```python
from build123d import *

# Parameters (mm, degrees)
F0_R     = 74.736194
F1_DEPTH = 25.4
F2_SIZE  = 5.08


with BuildPart() as f1:
    # F0 (on Top) → F1 (new body)
    with BuildSketch(Plane.XY):
        with Locations((-20.023532, 0)):
            Circle(F0_R)
        Polygon((-49.93894, 17.944667), (-38.893249, 41.878957), (14.034008, 41.878957), (0, 12.881645), (13.113534, 12.881645), (-11.739265, -19.337591), (7.130454, -19.337591), (-38.893249, -57.080124), (-29.228272, -17.496489), (-49.93894, -17.496489), (-31.529456, 17.944667), align=None, mode=Mode.SUBTRACT)
    extrude(amount=F1_DEPTH)

    # F2
    f2_edges = [f1.edges().sort_by_distance(p)[0] for p in [
        (-94.759726, 0, 25.4),
    ]]
    chamfer(f2_edges, length=F2_SIZE)


solid = f1.part
```
Design review of the part built by this model. Coordinates are the model's own, in mm. A direction names the side the tool comes from. Coordinates: 2 decimals unless noted, no trailing zeros. Order: outer loops, then holes, each group sorted by start corner. A loop starts at its lowest first (then second) coordinate and runs counter-clockwise, first axis right, second up. Notation, with made-up numbers: (24.25, 70) - (53.25, 70) arc R18 cw to (53.25, 104) - close; hole circle Ø7 at (16, 0.25). An arc over 180 degrees is marked (long way). Answer in a Markdown table with one row per item.
(1) Consider section A-A on z = 13.75. State the section outline as (x, y) points.
Checked values:
| item | result |
|---|---|
| outline | circle Ø149.47 at (-20.02, 0); hole (-49.94, -17.5) - (-29.23, -17.5) - (-38.89, -57.08) - (7.13, -19.34) - (-11.74, -19.34) - (13.11, 12.88) - (0, 12.88) - (14.03, 41.88) - (-38.89, 41.88) - (-49.94, 17.94) - (-31.53, 17.94) - close |
(2) Wall thickness on line 1 along Y through (x, z) = (-10, 8.25); line 2 along Y through (x, z) = (9, 11.75); line 3 along X through (y, z) = (21, 20.25): over which ranges is each line inside the solid? List them lowest first. Write a range as from..to.
Checked values:
| item | result |
|---|---|
| line 1 | -74.06..-33.39, -19.34..-17.08, 41.88..74.06 |
| line 2 | -68.87..7.55, 12.88..31.48, 41.88..68.87 |
| line 3 | -91.75..-48.53, 3.93..51.7 |
(3) Clearance check with flat-ended pins moving along their axes: pin 1 (1 mm diameter, centred on y = -14.5, z = 14.5, fed in from -X); pin 2 (14.5 mm diameter, centred on x = -43.5, z = 11, fed in from +Y); pin 3 (1 mm diameter, centred on y = 24, z = 9, fed in from -X). State where each tip first meets the part, or that it passes through.
Checked values:
| item | result |
|---|---|
| pin 1 | x = -93.44 |
| pin 2 | y = 72.95 |
| pin 3 | x = -90.97 |
(4) Consider section C-C on z = 22.75. State the section outline as (x, y) points.
Checked values:
| item | result |
|---|---|
| outline | circle Ø144.61 at (-20.02, 0); hole (-49.94, -17.5) - (-29.23, -17.5) - (-38.89, -57.08) - (7.13, -19.34) - (-11.74, -19.34) - (13.11, 12.88) - (0, 12.88) - (14.03, 41.88) - (-38.89, 41.88) - (-49.94, 17.94) - (-31.53, 17.94) - close |
(5) For faces 1 (the flat face through (0.861, -3.002, 12.522)), 2 (the conical face through (-75.496, -42.535, 25.153)), list the 3-axis set-ups (+Z, -Z, +X, -X, +Y, -Y) from which the entire face can be reached by the end or side of a thin tool; tool diameter is ignored.
Checked values:
| item | result |
|---|---|
| face 1 | +Z, -Z |
| face 2 | +Z |
(6) Consider section B-B on y = 0. State the section outline as (x, z) points, plus the area to 3 significant figures.
Checked values:
| item | result |
|---|---|
| outline | (-94.76, 0) - (-40.85, 0) - (-40.85, 25.4) - (-89.68, 25.4) - (-94.76, 20.32) - close; (3.18, 0) - (54.71, 0) - (54.71, 20.32) - (49.63, 25.4) - (3.18, 25.4) - close |
| area | 2,650 mm^2 |
